Verification items for the finished model (mm, model axes). Give positions to 0.01 mm unless a question says otherwise; leave off trailing zeros. Order: outer loops, then holes, each group sorted by start corner. A loop starts at its lowest first (then second) coordinate and runs counter-clockwise, first axis right, second up. Notation, with made-up numbers: (88.25, 73) -> (138.25, 73) arc R27 cw to (138.25, 91) -> close; hole circle Ø4 at (89, -26). An arc over 180 degrees is marked (long way). Return JSON: item names as keys, results as strings. Group by question number.
(1) Release check for a two-part mould opening along X. For faces 1 (the face through (65.393, 5, 12)), 2 (the face through (16, 5, 21.762)), 3 (the face through (62.256, 3.813, 11.902)), 4 (the face through (-4.99, 4.93, 19.158)) record: pulls with the +X half, pulls with the -X half, needs draft (parallel to the pull), parting line crosses it, or undercut.
(2) Thickness scan on line 1 along X through (y, z) = (8.25, 2.5); line 2 along X through (y, z) = (8.5, 9); line 3 along X through (y, z) = (5.75, 16.25). Record the ranges inside material, lowest first.
(3) Cross-section at C-C on x = 58. Enter the section's corners in (y, z).
(4) Cross-section at D-D on z = 12. Enter the section's corners in (x, y).
(5) Cross-section at A-A on y = 5. Enter the section's corners in (x, z).
(6) Cross-section at B-B on z = 3.5. Enter the section's corners in (x, y).
(7) Depth check by flat-ended pin: pin 1 Ø5 at (x, y) = (-3, 7.5) entering from -Z; pin 2 Ø5 at (x, z) = (53, 11) entering from -Y. Enter the tip coordinate at first touch or a pass-through.
from build123d import *

# Parameters (mm, degrees)
BOSS_EXTRUDE1_DEPTH = 10
SKETCH2_R           = 3.1
CUT_EXTRUDE1_DEPTH  = 70.110171815


with BuildPart() as part:
    # Sketch1 → Boss-Extrude1 (new body)
    with BuildSketch(Plane(origin=(0, 0, 0), x_dir=(1, 0, 0), z_dir=(0, 1, 0))):
        with BuildLine():
            Line((12.792781316, -1.762208068), (17.992781316, -1.762208068))
            ThreePointArc((17.992781316, -1.762208068), (35.392781316, -19.162208068), (52.792781316, -1.762208068))
            Line((52.792781316, -1.762208068), (65.392781316, -1.762208068))
            Line((65.392781316, -1.762208068), (65.392781316, -21.762208068))
            Line((65.392781316, -21.762208068), (-34.607218684, -21.762208068))
            Line((-34.607218684, -21.762208068), (-34.607218684, -1.762208068))
            Line((-34.607218684, -1.762208068), (-22.007218684, -1.762208068))
            ThreePointArc((-22.007218684, -1.762208068), (-4.607218684, -19.162208068), (12.792781316, -1.762208068))
        make_face()
    extrude(amount=BOSS_EXTRUDE1_DEPTH)

    # Sketch2 → Cut-Extrude1 (cut, through all)
    with BuildSketch(Plane.XY.offset(21.762208068)):
        with Locations((-28.607218684, 5)):
            Circle(SKETCH2_R)
        with Locations((59.392781316, 5)):
            Circle(SKETCH2_R)
    extrude(amount=-CUT_EXTRUDE1_DEPTH, mode=Mode.SUBTRACT)


solid = part.part
Verdict:
{
 "1": {"face 1": "pulls with the +X half", "face 2": "needs draft", "face 3": "undercut", "face 4": "undercut"},
 "2": {"line 1": "-34.61 to -21.99, 12.78 to 18.01, 52.78 to 65.39", "line 2": "-34.61 to -20.43, 11.22 to 19.57, 51.22 to 65.39", "line 3": "-34.61 to -31.62, -25.6 to -14.24, 5.03 to 25.76, 45.03 to 56.38, 62.4 to 65.39"},
 "3": {"outline": "(0, 1.76) -> (2.23, 1.76) -> (2.23, 21.76) -> (0, 21.76) -> close; (7.77, 1.76) -> (10, 1.76) -> (10, 21.76) -> (7.77, 21.76) -> close"},
 "4": {"outline": "(-34.61, 0) -> (-18.68, 0) -> (-18.68, 10) -> (-34.61, 10) -> close; (9.46, 0) -> (21.32, 0) -> (21.32, 10) -> (9.46, 10) -> close; (49.46, 0) -> (65.39, 0) -> (65.39, 10) -> (49.46, 10) -> close; hole circle Ø6.2 at (-28.61, 5); hole circle Ø6.2 at (59.39, 5)"},
 "5": {"outline": "(-34.61, 1.76) -> (-31.71, 1.76) -> (-31.71, 21.76) -> (-34.61, 21.76) -> close; (-25.51, 1.76) -> (-22.01, 1.76) arc R17.4 cw to (12.79, 1.76) -> (17.99, 1.76) arc R17.4 cw to (52.79, 1.76) -> (56.29, 1.76) -> (56.29, 21.76) -> (-25.51, 21.76) -> close; (62.49, 1.76) -> (65.39, 1.76) -> (65.39, 21.76) -> (62.49, 21.76) -> close"},
 "6": {"outline": "(-34.61, 0) -> (-21.92, 0) -> (-21.92, 10) -> (-34.61, 10) -> close; (12.71, 0) -> (18.08, 0) -> (18.08, 10) -> (12.71, 10) -> close; (52.71, 0) -> (65.39, 0) -> (65.39, 10) -> (52.71, 10) -> close; hole circle Ø6.2 at (-28.61, 5); hole circle Ø6.2 at (59.39, 5)"},
 "7": {"pin 1": "z = 18.67", "pin 2": "y = 0"}
}
